Autodesk Fusion 360 part; units mm, degrees
sketch "スケッチ1" plane through (0, 0, 0) normal (1, 0, 0) x (0, 1, 0)
  line L0 (0, 0) -> (46, 0)
  line L1 (46, 0) -> (46, 44)
  line L2 (46, 44) -> (0, 44)
  line L3 (0, 44) -> (0, 0)
  dimension "d1" = 46
  dimension "d2" = 44
extrude "押し出し1" add sketch "スケッチ1" along normal blind 2
sketch "スケッチ2" plane through (2, 0, 0) normal (1, 0, 0) x (0, 1, 0)
  line L0 (0, 44) -> (0, 0)
  line L1 (0, 0) -> (46, 0)
  line L2 (46, 0) -> (46, 44)
  line L3 (46, 44) -> (0, 44)
  line L4 (0, 0) -> (8, 0)
  line L5 (8, 0) -> (8, 2)
  line L6 (8, 2) -> (0, 2)
  line L7 (0, 2) -> (0, 0)
  line L8 (14, 0) -> (20, 0)
  line L9 (20, 0) -> (20, 2)
  line L10 (20, 2) -> (14, 2)
  line L11 (14, 2) -> (14, 0)
  line L12 (26, 0) -> (32, 0)
  line L13 (32, 0) -> (32, 2)
  line L14 (32, 2) -> (26, 2)
  line L15 (26, 2) -> (26, 0)
  line L16 (46, 0) -> (38, 0)
  line L17 (38, 0) -> (38, 2)
  line L18 (38, 2) -> (46, 2)
  line L19 (46, 2) -> (46, 0)
  line L20 (32, 42) -> (32, 44)
  line L21 (32, 44) -> (26, 44)
  line L22 (20, 42) -> (20, 44)
  line L23 (38, 42) -> (38, 44)
  line L24 (38, 44) -> (46, 44)
  line L25 (46, 44) -> (46, 42)
  line L26 (0, 42) -> (8, 42)
  line L27 (26, 44) -> (26, 42)
  line L28 (8, 42) -> (8, 44)
  line L29 (8, 44) -> (0, 44)
  line L30 (0, 44) -> (0, 42)
  line L31 (20, 44) -> (14, 44)
  line L32 (26, 42) -> (32, 42)
  line L33 (46, 42) -> (38, 42)
  line L34 (14, 42) -> (20, 42)
  line L35 (14, 44) -> (14, 42)
  point P0 (0, 42)
  dimension "d5" = 8
  dimension "d6" = 2
  dimension "d7" = 6
  dimension "d8" = 2
  dimension "d9" = 6
  dimension "d10" = 6
  dimension "d11" = 2
  dimension "d12" = 6
  dimension "d13" = 6
  dimension "d14" = 2
extrude "押し出し2" cut sketch "スケッチ2" against normal blind 2 contours L0 L3 L26 L28 L29 L30 | L0 L1 L4 L5 L6 L7 | L3 L22 L31 L34 L35 | L3 L20 L21 L27 L32 | L1 L8 L9 L10 L11 | L2 L3 L23 L24 L25 L33 | L1 L12 L13 L14 L15 | L1 L2 L16 L17 L18 L19
sketch "スケッチ3" plane through (2, 0, 0) normal (1, 0, 0) x (0, 1, 0)
  line L0 (8, 2) -> (8, 0)
  line L1 (8, 0) -> (14, 0)
  line L2 (14, 0) -> (14, 2)
  line L3 (14, 2) -> (20, 2)
  line L4 (20, 2) -> (20, 0)
  line L5 (20, 0) -> (26, 0)
  line L6 (26, 0) -> (26, 2)
  line L7 (26, 2) -> (32, 2)
  line L8 (32, 2) -> (32, 0)
  line L9 (32, 0) -> (38, 0)
  line L10 (38, 0) -> (38, 2)
  line L11 (38, 2) -> (46, 2)
  line L12 (46, 2) -> (46, 42)
  line L13 (46, 42) -> (38, 42)
  line L14 (38, 42) -> (38, 44)
  line L15 (38, 44) -> (32, 44)
  line L16 (32, 44) -> (32, 42)
  line L17 (32, 42) -> (26, 42)
  line L18 (26, 42) -> (26, 44)
  line L19 (26, 44) -> (20, 44)
  line L20 (20, 44) -> (20, 42)
  line L21 (20, 42) -> (14, 42)
  line L22 (14, 42) -> (14, 44)
  line L23 (14, 44) -> (8, 44)
  line L24 (8, 44) -> (8, 42)
  line L25 (8, 42) -> (0, 42)
  line L26 (0, 42) -> (0, 2)
  line L27 (0, 2) -> (8, 2)
  line L28 (0, 44) -> (2, 44)
  line L29 (2, 44) -> (2, 37)
  line L30 (2, 37) -> (0, 37)
  line L31 (0, 37) -> (0, 44)
  line L32 (2, 31) -> (0, 31)
  line L33 (0, 31) -> (0, 25)
  line L34 (0, 25) -> (2, 25)
  line L35 (2, 25) -> (2, 31)
  line L36 (2, 19) -> (0, 19)
  line L37 (0, 19) -> (0, 13)
  line L38 (0, 13) -> (2, 13)
  line L39 (2, 13) -> (2, 19)
  line L40 (2, 7) -> (0, 7)
  line L41 (0, 7) -> (0, 0)
  line L42 (0, 0) -> (2, 0)
  line L43 (2, 0) -> (2, 7)
  line L44 (46, 31) -> (44, 31)
  line L45 (46, 13) -> (46, 19)
  line L46 (44, 44) -> (46, 44)
  line L47 (44, 0) -> (46, 0)
  line L48 (44, 7) -> (44, 0)
  line L49 (44, 25) -> (46, 25)
  line L50 (46, 37) -> (44, 37)
  line L51 (44, 37) -> (44, 44)
  line L52 (44, 13) -> (46, 13)
  line L53 (44, 31) -> (44, 25)
  line L54 (46, 19) -> (44, 19)
  line L55 (44, 19) -> (44, 13)
  line L56 (46, 25) -> (46, 31)
  line L57 (46, 7) -> (44, 7)
  line L58 (46, 0) -> (46, 7)
  line L59 (46, 44) -> (46, 37)
  point P0 (44, 0)
  dimension "d21" = 2
  dimension "d22" = 7
  dimension "d23" = 2
  dimension "d24" = 6
  dimension "d25" = 6
  dimension "d26" = 6
  dimension "d27" = 6
  dimension "d28" = 2
  dimension "d29" = 6
  dimension "d30" = 7
  dimension "d31" = 2
extrude "押し出し3" cut sketch "スケッチ3" against normal blind 2 contours L27 L41 L42 L43 | L26 L27 L40 L41 L43 | L26 L36 L37 L38 L39 | L26 L32 L33 L34 L35 | L25 L26 L29 L30 L31 | L25 L28 L29 L31 | L11 L12 L48 L57 L58 | L11 L47 L48 L58 | L12 L45 L52 L54 L55 | L12 L44 L49 L53 L56 | L12 L13 L50 L51 L59 | L13 L46 L51 L59
sketch "スケッチ4" plane through (2, 0, 0) normal (1, 0, 0) x (0, 1, 0)
  line L0 (44, 19) -> (46, 19)
  line L1 (46, 19) -> (46, 25)
  line L2 (46, 25) -> (44, 25)
  line L3 (44, 25) -> (44, 31)
  line L4 (44, 31) -> (46, 31)
  line L5 (46, 31) -> (46, 37)
  line L6 (46, 37) -> (44, 37)
  line L7 (44, 37) -> (44, 42)
  line L8 (44, 42) -> (38, 42)
  line L9 (38, 42) -> (38, 44)
  line L10 (38, 44) -> (32, 44)
  line L11 (32, 44) -> (32, 42)
  line L12 (32, 42) -> (26, 42)
  line L13 (26, 42) -> (26, 44)
  line L14 (26, 44) -> (20, 44)
  line L15 (20, 44) -> (20, 42)
  line L16 (20, 42) -> (14, 42)
  line L17 (14, 42) -> (14, 44)
  line L18 (14, 44) -> (8, 44)
  line L19 (8, 44) -> (8, 42)
  line L20 (8, 42) -> (2, 42)
  line L21 (2, 42) -> (2, 37)
  line L22 (2, 37) -> (0, 37)
  line L23 (0, 37) -> (0, 31)
  line L24 (0, 31) -> (2, 31)
  line L25 (2, 31) -> (2, 25)
  line L26 (2, 25) -> (0, 25)
  line L27 (0, 25) -> (0, 19)
  line L28 (0, 19) -> (2, 19)
  line L29 (2, 19) -> (2, 13)
  line L30 (2, 13) -> (0, 13)
  line L31 (0, 13) -> (0, 7)
  line L32 (0, 7) -> (2, 7)
  line L33 (2, 7) -> (2, 2)
  line L34 (2, 2) -> (8, 2)
  line L35 (8, 2) -> (8, 0)
  line L36 (8, 0) -> (14, 0)
  line L37 (14, 0) -> (14, 2)
  line L38 (14, 2) -> (20, 2)
  line L39 (20, 2) -> (20, 0)
  line L40 (20, 0) -> (26, 0)
  line L41 (26, 0) -> (26, 2)
  line L42 (26, 2) -> (32, 2)
  line L43 (32, 2) -> (32, 0)
  line L44 (32, 0) -> (38, 0)
  line L45 (38, 0) -> (38, 2)
  line L46 (38, 2) -> (44, 2)
  line L47 (44, 2) -> (44, 7)
  line L48 (44, 7) -> (46, 7)
  line L49 (46, 7) -> (46, 13)
  line L50 (46, 13) -> (44, 13)
  line L51 (44, 13) -> (44, 19)
  line L52 (10, 15) -> (12, 15)
  line L53 (12, 15) -> (12, 25)
  line L54 (12, 25) -> (10, 25)
  line L55 (10, 25) -> (10, 15)
  line L56 (15, 15) -> (17, 15)
  line L57 (17, 15) -> (17, 25)
  line L58 (17, 25) -> (15, 25)
  line L59 (15, 25) -> (15, 15)
  line L60 (20, 15) -> (22, 15)
  line L61 (22, 15) -> (22, 25)
  line L62 (22, 25) -> (20, 25)
  line L63 (20, 25) -> (20, 15)
  line L64 (25, 15) -> (27, 15)
  line L65 (27, 15) -> (27, 25)
  line L66 (27, 25) -> (25, 25)
  line L67 (25, 25) -> (25, 15)
  line L68 (30, 15) -> (32, 15)
  line L69 (32, 15) -> (32, 25)
  line L70 (32, 25) -> (30, 25)
  line L71 (30, 25) -> (30, 15)
  line L72 (35, 15) -> (37, 15)
  line L73 (37, 15) -> (37, 25)
  line L74 (37, 25) -> (35, 25)
  line L75 (35, 25) -> (35, 15)
extrude "押し出し4" cut sketch "スケッチ4" against normal blind 2 contours L52 L53 L54 L55 | L56 L57 L58 L59 | L60 L61 L62 L63 | L64 L65 L66 L67 | L68 L69 L70 L71 | L72 L73 L74 L75
Input: part model. Units: mm. Frame: model coordinates. A direction names the side the tool comes from. Round coordinates to 2 decimals unless told otherwise and drop trailing zeros. Order: outer loops, then holes, each group sorted by start corner. A loop starts at its lowest first (then second) coordinate and runs counter-clockwise, first axis right, second up. Notation, with made-up numbers: (76, 79.5) - (117, 79.5) arc R20 ccw to (117, 118.5) - close; hole circle Ø10 at (-10, 75). An arc over 180 degrees is marked (long way). Use a Markdown table: item, result.
1. Material intervals for probe 1 along Y at (x, z) = (1.45, 42.5); probe 2 along Z at (x, y) = (0.8, 44.5); probe 3 along Z at (x, y) = (0.1, 30.5), sorted ascending.
Evaluation:
| item | result |
|---|---|
| probe 1 | 8 to 14, 20 to 26, 32 to 38 |
| probe 2 | 7 to 13, 19 to 25, 31 to 37 |
| probe 3 | 2 to 15, 25 to 42 |
2. Mould query, pull axis Y, two halves, no side actions, for faces 1 (the face through (1, 2, 16)), 2 (the face through (1, 36, 25)), 3 (the face through (1, 1, 19)). Classes: +Y half, -Y half, draft (parallel to the pull), parting line (faces both ways), or undercut.
Evaluation:
| item | result |
|---|---|
| face 1 | -Y half |
| face 2 | undercut |
| face 3 | draft |
3. Section D-D on z = 39. Return the cut outline in (x, y).
Evaluation:
| item | result |
|---|---|
| outline | (0, 2) - (2, 2) - (2, 44) - (0, 44) - close |
4. Section A-A on z = 20. Return the cut outline in (x, y).
Evaluation:
| item | result |
|---|---|
| outline | (0, 0) - (2, 0) - (2, 10) - (0, 10) - close; (0, 12) - (2, 12) - (2, 15) - (0, 15) - close; (0, 17) - (2, 17) - (2, 20) - (0, 20) - close; (0, 22) - (2, 22) - (2, 25) - (0, 25) - close; (0, 27) - (2, 27) - (2, 30) - (0, 30) - close; (0, 32) - (2, 32) - (2, 35) - (0, 35) - close; (0, 37) - (2, 37) - (2, 46) - (0, 46) - close |
5. Section B-B on y = 5.5. Return the cut outline in (x, z), then the cut area to 3 significant figures.
Evaluation:
| item | result |
|---|---|
| outline | (0, 2) - (2, 2) - (2, 42) - (0, 42) - close |
| area | 80.0 mm^2 |
6. Access query for faces 4 (the face through (1, 45, 37)), 5 (the face through (1, 8, 43)), 6 (the face through (1, 21, 25)), 7 (the face through (1, 17, 2)). Directions: +Z, -Z, +X, -X, +Y, -Y. A direction counts if a zero-diameter tool reaches every point of the face in a straight line with its end or side. Return the directions, or none.
Evaluation:
| item | result |
|---|---|
| face 4 | +Z, +X, -X, +Y |
| face 5 | +Z, +X, -X, -Y |
| face 6 | +X, -X |
| face 7 | -Z, +X, -X |
7. First-contact query: pin 1 (0.6 mm diameter, centred on x = 1, z = 43, fed in from +Y); pin 2 (0.6 mm diameter, centred on x = 1, z = 40.5, fed in from -Y); pin 3 (0.6 mm diameter, centred on x = 1.5, y = 31, fed in from -Z). Flat tips, straight axial feed; report the tip coordinate or a pass-through.
Evaluation:
| item | result |
|---|---|
| pin 1 | y = 38 |
| pin 2 | y = 2 |
| pin 3 | z = 2 |
8. Section C-C on x = 1.35. State how many separate pieces and enclosed holes the cut face has, then the cut area to 3 significant figures.
Evaluation:
| item | result |
|---|---|
| separate pieces | 1 |
| enclosed holes | 6 |
| area | 1,700 mm^2 |
